Here's how the part is built. I have some questions about the finished solid (model axes, mm). A direction names the side the tool comes from. Coordinates: 2 decimals unless noted, no trailing zeros. Write each loop counter-clockwise with the first axis right and the second up, starting at its lowest first coordinate (ties: lowest second). Pieces come first, ordered by that corner, then holes.
```python
from build123d import *

# Parameters (mm, degrees)
SKETCH_1_W          = 56
SKETCH_1_H          = 60
EXTRUDE_1_DEPTH     = 5
SKETCH_2_R          = 2
CUT_EXTRUDE_1_DEPTH = 5
SKETCH_3_W          = 56
SKETCH_3_H          = 4.7
EXTRUDE_2_DEPTH     = 30
SKETCH_4_R          = 1.55
CUT_EXTRUDE_2_DEPTH = 40
SKETCH_5_W          = 25
SKETCH_5_H          = 24
EXTRUDE_3_DEPTH     = 4.3
EXTRUDE_4_DEPTH     = 15


with BuildPart() as part:
    # 草图1 → 凸台-拉伸1 (new body)
    with BuildSketch(Plane.XY):
        Rectangle(SKETCH_1_W, SKETCH_1_H)
    extrude(amount=EXTRUDE_1_DEPTH)

    # 草图2 → 切除-拉伸1 (cut)
    with BuildSketch(Plane.XY.offset(5)):
        with Locations((-16, -23.4)):
            Circle(SKETCH_2_R)
        with Locations((-16, -9.4)):
            Circle(SKETCH_2_R)
    cut_extrude_1 = extrude(amount=-CUT_EXTRUDE_1_DEPTH, mode=Mode.SUBTRACT)

    # 镜向1: 切除-拉伸1 across plane
    add(cut_extrude_1.mirror(Plane(origin=(0, 0, 0), x_dir=(0, 0, 1), z_dir=(1, 0, 0))), mode=Mode.SUBTRACT)

    # 草图3 → 凸台-拉伸2 (add)
    with BuildSketch(Plane.XY.offset(5)):
        with Locations((0, 27.65)):
            Rectangle(SKETCH_3_W, SKETCH_3_H)
    extrude(amount=EXTRUDE_2_DEPTH)

    # 草图4 → 切除-拉伸2 (cut)
    with BuildSketch(Plane(origin=(0, 30, 0), x_dir=(1, 0, 0), z_dir=(0, 1, 0))):
        with Locations(Location((-7, -27, 0), (0, 0, 270))):
            Circle(SKETCH_4_R)
    extrude(amount=-CUT_EXTRUDE_2_DEPTH, mode=Mode.SUBTRACT)

    # 草图5 → 凸台-拉伸3 (add)
    with BuildSketch(Plane.XY.offset(5)):
        with Locations((-15.5, 13.3)):
            Rectangle(SKETCH_5_W, SKETCH_5_H)
    extrude(amount=EXTRUDE_3_DEPTH)

    # 草图6 → 凸台-拉伸4 (add)
    with BuildSketch(Plane.ZY.offset(28)):
        Polygon((0, 26.5), (0, -3.5), (9.5, -3.5), (9.5, 31.5), (0, 31.5), align=None)
    extrude_4 = extrude(amount=EXTRUDE_4_DEPTH)

    # 镜向2: 凸台-拉伸4 across plane
    add(extrude_4.mirror(Plane(origin=(0, 0, 0), x_dir=(0, 0, 1), z_dir=(1, 0, 0))))


solid = part.part
```
1) We'd pull the mould along Y, two halves only. Please class faces 1 (the face through (-17.474, -8.048, 2.535)), 2 (the face through (-35, -3.5, 5)), 3 (the face through (6, -8, 5)), 4 (the face through (-17.6, -24.6, 2.5)): pulls with the +Y half, pulls with the -Y half, needs draft (parallel to the pull), parting line crosses it, or undercut.
Values follow:
face 1: undercut
face 2: pulls with the -Y half
face 3: needs draft
face 4: undercut
2) Imagine slicing it at A-A on x = -7. Please give me the cut outline in (y, z).
Values follow:
outline: (-30, 0) - (30, 0) - (30, 25.45) - (25.3, 25.45) - (25.3, 9.3) - (1.3, 9.3) - (1.3, 5) - (-30, 5) - close; (25.3, 28.55) - (30, 28.55) - (30, 35) - (25.3, 35) - close
3) On a 3-axis mill with a long thin cutter (end or side, diameter ignored), from which of +Z, -Z, +X, -X, +Y, -Y can I reach the whole of each face in a straight line? I mean faces 5 (the face through (-3, 13, 7)), 6 (the face through (0, 30, 17)), 7 (the face through (35, -3.5, 5)). Say none if no direction works.
Values follow:
face 5: +Z, -Y
face 6: +Z, -Z, +Y
face 7: +Z, -Z, +X, -Y
4) Will these pins go through, and if not, where does the flat tip stop? pin 1 (15 mm diameter, centred on x = -6, z = 14.5, fed in from -Y); pin 2 (3 mm diameter, centred on x = 16, y = -23.4, fed in from +Z); pin 3 (12 mm diameter, centred on x = -0.5, z = 5, fed in from +Y); pin 4 (12 mm diameter, centred on x = -36, y = 10.5, fed in from +Z).
Values follow:
pin 1: stops at y = 1.3
pin 2: passes through
pin 3: stops at y = 30
pin 4: stops at z = 9.5
5) I need wall thicknesses on probe 1 along Y at (x, z) = (16, 2.65); probe 2 along X at (y, z) = (-9, 3); probe 3 along X at (y, z) = (28, 27). Which ranges of each line are inside material? Lowest first, please.
Values follow:
probe 1: y = -30 to -25.4, -21.4 to -11.4, -7.4 to 30
probe 2: x = -28 to -17.96, -14.04 to 14.04, 17.96 to 28
probe 3: x = -28 to -8.55, -5.45 to 28
6) Imagine slicing it at C-C on y = -23.4. Please give me the cut outline in (x, z).
Values follow:
outline: (-28, 0) - (-18, 0) - (-18, 5) - (-28, 5) - close; (-14, 0) - (14, 0) - (14, 5) - (-14, 5) - close; (18, 0) - (28, 0) - (28, 5) - (18, 5) - close
7) Imagine slicing it at D-D on x = -26. Please give me the cut outline in (y, z).
Values follow:
outline: (-30, 0) - (30, 0) - (30, 35) - (25.3, 35) - (25.3, 9.3) - (1.3, 9.3) - (1.3, 5) - (-30, 5) - close
8) Imagine slicing it at B-B on z = 6. Please give me the cut outline in (x, y), then the cut area to 3 significant figures.
Values follow:
outline: (-43, -3.5) - (-28, -3.5) - (-28, 1.3) - (-3, 1.3) - (-3, 25.3) - (28, 25.3) - (28, -3.5) - (43, -3.5) - (43, 31.5) - (28, 31.5) - (28, 30) - (-28, 30) - (-28, 31.5) - (-43, 31.5) - close
area: 1,910 mm2
